Geometry: final body of the model. Coordinates: model frame, mm. Face numbers are marked on the shaded views. A direction names the side the tool comes from. Coordinates: 2 decimals unless noted, no trailing zeros. Order: outer loops, then holes, each group sorted by start corner. A loop starts at its lowest first (then second) coordinate and runs counter-clockwise, first axis right, second up. Notation, with made-up numbers: M 37.25,86.25 L 54.25,86.25 A26 cw 54.25,123.25 Z; hole C 64.25,18 d11. An arc over 180 degrees is marked long. Use CSV: the item, a comma, the result in double quotes. Start each with the question number.
1. Set-up query: the marked faces 4, 5, 6, 7 and 8. Return all of +Z, -Z, +X, -X, +Y, -Y with unobstructed straight access to the full face (end or side cutting, diameter ignored); none if empty.
2. Section query A-A on x = 68. Return the cut outline in (y, z), and give its area (3 significant figures).
3. Material intervals for line 1 (Z direction, x = 68, y = 48.2); line 2 (Y direction, x = 0, z = -2.5); line 3 (X direction, y = 21.5, z = -3), sorted ascending.
4. First-contact query: P1, Ø18, axis at x = 70.5, z = -8.5, coming from the -Y side; P2, Ø1, axis at y = 24, z = 19, coming from the -X side; P3, Ø1.5, axis at x = 27, z = -16, coming from the +Y side; P4, Ø4.5, axis at x = -68, z = 0, coming from the -Y side. Flat tips, straight axial feed; report the tip coordinate or a pass-through.
5. Section query D-D on z = 18. Return the cut outline in (x, y), and give its area (3 significant figures).
6. Pull-direction query (Y, two-part tool) for the marked faces 1, 2 and 3; classes: pulls with the +Y half, pulls with the -Y half, needs draft (parallel to the pull), parting line crosses it, or undercut.
7. Section query B-B on z = 0. Return the cut outline in (x, y), and give its area (3 significant figures).
8. Section query C-C on y = 41. Return the cut outline in (x, z), and give its area (3 significant figures).
from build123d import *

# Parameters (mm, degrees)
BOSS_EXTRUDE1_DEPTH = 25
BOSS_EXTRUDE3_START = -5
BOSS_EXTRUDE3_DEPTH = 5
HOLE1_D             = 14
HOLE2_D             = 5
FILLET1_R           = 10


with BuildPart() as part:
    # Sketch1 → Boss-Extrude1 (new, symmetric)
    with BuildSketch(Plane.XY):
        with BuildLine():
            Line((-35, 0), (-35, 29.811196065))
            Line((-35, 29.811196065), (-57.5, 45))
            Line((-57.5, 45), (-80, 45))
            Line((-80, 45), (-80, 51))
            Line((-80, 51), (-55.664377376, 51))
            Line((-55.664377376, 51), (-29, 33))
            Line((-29, 33), (-29, 25))
            Line((-29, 25), (-10.583005244, 25))
            ThreePointArc((-10.583005244, 25), (0, 33), (10.583005244, 25))
            Line((10.583005244, 25), (29, 25))
            Line((29, 25), (29, 33))
            Line((29, 33), (55.664377376, 51))
            Line((55.664377376, 51), (80, 51))
            Line((80, 51), (80, 45))
            Line((80, 45), (57.5, 45))
            Line((57.5, 45), (35, 29.811196065))
            Line((35, 29.811196065), (35, 0))
            Line((35, 0), (-35, 0))
        make_face()
    extrude(amount=BOSS_EXTRUDE1_DEPTH, both=True)

    # Sketch2 → Boss-Extrude3 (add)
    with BuildSketch(Plane.XY.offset(25).offset(BOSS_EXTRUDE3_START)):
        with BuildLine():
            Line((55.664377376, 51), (29, 33))
            Line((29, 33), (29, 25))
            Line((29, 25), (10.583005244, 25))
            ThreePointArc((10.583005244, 25), (0, 33), (-10.583005244, 25))
            Line((-10.583005244, 25), (-29, 25))
            Line((-29, 25), (-29, 33))
            Line((-29, 33), (-55.664377376, 51))
            Line((-55.664377376, 51), (0, 33.529077086))
            Line((0, 33.529077086), (55.664377376, 51))
        make_face()
    extrude(amount=-BOSS_EXTRUDE3_DEPTH)

    # Hole1 (through all)
    with Locations(Plane.XY.offset(25)):
        with Locations((0, 22)):
            Hole(HOLE1_D / 2)

    # Hole2 (through all)
    with Locations(Plane(origin=(0, 51, 0), x_dir=(1, 0, 0), z_dir=(0, 1, 0))):
        with Locations((68, 0)):
            hole2 = Hole(HOLE2_D / 2)

    # Mirror1: Hole2 across plane
    add(hole2.mirror(Plane(origin=(0, 0, 0), x_dir=(0, 0, 1), z_dir=(1, 0, 0))), mode=Mode.SUBTRACT)

    # Fillet1
    fillet1_edges = [part.edges().sort_by_distance(p)[0] for p in [
        (-80, 48, -25),
        (80, 48, 25),
        (80, 48, -25),
        (-80, 48, 25),
    ]]
    fillet(fillet1_edges, radius=FILLET1_R)


solid = part.part
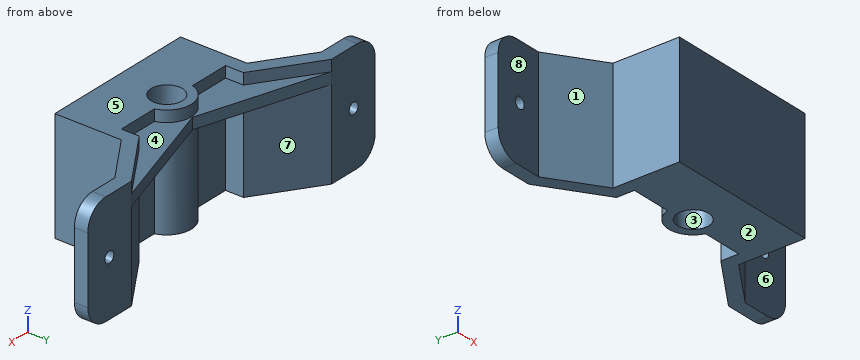
Results list:
1,face 4,"+Z, +Y"
1,face 5,"+Z, +X, -X, +Y, -Y"
1,face 6,"+Z, -Z, +X, -Y"
1,face 7,"-Z, +Y"
1,face 8,"+Z, -Z, -X, -Y"
2,outline,"M 45,-25 L 51,-25 L 51,-2.5 L 45,-2.5 Z; M 45,2.5 L 51,2.5 L 51,25 L 45,25 Z"
2,area,"270 mm²"
3,line 1,"z = -25 to -2.5, 2.5 to 25"
3,line 2,"y = 0 to 15, 29 to 33"
3,line 3,"x = -35 to -6.98, 6.98 to 35"
4,P1,"stops at y = 45"
4,P2,"stops at x = -35"
4,P3,"stops at y = 25"
4,P4,"passes through"
5,outline,"M -79.54,45 L -57.5,45 L -35,29.81 L -35,0 L 35,0 L 35,29.81 L 57.5,45 L 79.54,45 L 79.54,51 L 55.66,51 L 0,33.53 L -55.66,51 L -79.54,51 Z; hole C 0,22 d14"
5,area,"3,320 mm²"
6,face 1,"pulls with the -Y half"
6,face 2,"needs draft"
6,face 3,"undercut"
7,outline,"M -80,45 L -70.5,45 L -70.5,51 L -80,51 Z; M -65.5,45 L -57.5,45 L -35,29.81 L -35,0 L 35,0 L 35,29.81 L 57.5,45 L 65.5,45 L 65.5,51 L 55.66,51 L 29,33 L 29,25 L 10.58,25 A11 ccw -10.58,25 L -29,25 L -29,33 L -55.66,51 L -65.5,51 Z; M 70.5,45 L 80,45 L 80,51 L 70.5,51 Z; hole C 0,22 d14"
7,area,"2,370 mm²"
8,outline,"M -51.57,-25 L -40.85,-25 L -40.85,15 L -23.8,15 L -23.8,20 L -40.85,20 L -40.85,25 L -51.57,25 Z; M 23.8,15 L 40.85,15 L 40.85,-25 L 51.57,-25 L 51.57,25 L 40.85,25 L 40.85,20 L 23.8,20 Z"
8,area,"1,240 mm²"
